from build123d import *

# Parameters (mm, degrees)
CHAMFER1_SIZE                                        = 2.5
CHAMFER2_SIZE                                        = 1.5
CSK_FOR_M10_COUNTERSUNK_FLAT_HEAD_SCREW1_D           = 11
CSK_FOR_M10_COUNTERSUNK_FLAT_HEAD_SCREW1_DEPTH       = 10.695266595
CSK_FOR_M10_COUNTERSUNK_FLAT_HEAD_SCREW1_CSINK_D     = 14
CSK_FOR_M10_COUNTERSUNK_FLAT_HEAD_SCREW1_CSINK_ANGLE = 90
CSK_FOR_M10_COUNTERSUNK_FLAT_HEAD_SCREW1_TIP         = 3.304733405
CSK_FOR_M10_COUNTERSUNK_FLAT_HEAD_SCREW2_D           = 11
CSK_FOR_M10_COUNTERSUNK_FLAT_HEAD_SCREW2_DEPTH       = 10.695266595
CSK_FOR_M10_COUNTERSUNK_FLAT_HEAD_SCREW2_CSINK_D     = 14
CSK_FOR_M10_COUNTERSUNK_FLAT_HEAD_SCREW2_CSINK_ANGLE = 90
CSK_FOR_M10_COUNTERSUNK_FLAT_HEAD_SCREW2_TIP         = 3.304733405


with BuildPart() as part:
    # Sketch1 → Revolve1 (revolve)
    with BuildSketch(Plane.XY):
        Polygon((0, 0), (0, 14.7), (17, 14.7), (17, 37.5), (109.5, 37.5), (109.5, 35), (128.5, 35), (141.5, 35), (141.5, 33), (257, 33), (257, 0), align=None)
    revolve(axis=Axis((0, 0, 0), (1, 0, 0)))

    # Chamfer1
    chamfer1_edges = [part.edges().sort_by_distance(p)[0] for p in [
        (17, -37.5, 0),
        (257, -33, 0),
    ]]
    chamfer(chamfer1_edges, length=CHAMFER1_SIZE)

    # Chamfer2
    chamfer2_edges = [part.edges().sort_by_distance(p)[0] for p in [
        (0, -14.7, 0),
    ]]
    chamfer(chamfer2_edges, length=CHAMFER2_SIZE)

    # CSK for M10 Countersunk Flat Head Screw1
    with Locations(Plane.ZY):
        with Locations((0, 0)):
            CounterSinkHole(CSK_FOR_M10_COUNTERSUNK_FLAT_HEAD_SCREW1_D / 2, CSK_FOR_M10_COUNTERSUNK_FLAT_HEAD_SCREW1_CSINK_D / 2, depth=CSK_FOR_M10_COUNTERSUNK_FLAT_HEAD_SCREW1_DEPTH, counter_sink_angle=CSK_FOR_M10_COUNTERSUNK_FLAT_HEAD_SCREW1_CSINK_ANGLE)
            with Locations((0, 0, -(CSK_FOR_M10_COUNTERSUNK_FLAT_HEAD_SCREW1_DEPTH + CSK_FOR_M10_COUNTERSUNK_FLAT_HEAD_SCREW1_TIP / 2))):  # 118° drill point
                Cone(0, CSK_FOR_M10_COUNTERSUNK_FLAT_HEAD_SCREW1_D / 2, CSK_FOR_M10_COUNTERSUNK_FLAT_HEAD_SCREW1_TIP, mode=Mode.SUBTRACT)

    # CSK for M10 Countersunk Flat Head Screw2
    with Locations(Plane(origin=(257, 0, 0), x_dir=(0, 0, -1), z_dir=(1, 0, 0))):
        with Locations((0, 0)):
            CounterSinkHole(CSK_FOR_M10_COUNTERSUNK_FLAT_HEAD_SCREW2_D / 2, CSK_FOR_M10_COUNTERSUNK_FLAT_HEAD_SCREW2_CSINK_D / 2, depth=CSK_FOR_M10_COUNTERSUNK_FLAT_HEAD_SCREW2_DEPTH, counter_sink_angle=CSK_FOR_M10_COUNTERSUNK_FLAT_HEAD_SCREW2_CSINK_ANGLE)
            with Locations((0, 0, -(CSK_FOR_M10_COUNTERSUNK_FLAT_HEAD_SCREW2_DEPTH + CSK_FOR_M10_COUNTERSUNK_FLAT_HEAD_SCREW2_TIP / 2))):  # 118° drill point
                Cone(0, CSK_FOR_M10_COUNTERSUNK_FLAT_HEAD_SCREW2_D / 2, CSK_FOR_M10_COUNTERSUNK_FLAT_HEAD_SCREW2_TIP, mode=Mode.SUBTRACT)


solid = part.part
Input: part model. Units: mm. Frame: model coordinates. A direction names the side the tool comes from. Give positions to 0.01 mm unless a question says otherwise; leave off trailing zeros. Write each loop counter-clockwise with the first axis right and the second up, starting at its lowest first coordinate (ties: lowest second). Pieces come first, ordered by that corner, then holes.
Q1. Material intervals for probe 1 along Z at (x, y) = (249, 0); probe 2 along Z at (x, y) = (7, 0); probe 3 along X at (y, z) = (26, -15), sorted ascending.
Q2. Section B-B, the plane x = 218. Output: boundary loops of the cut face in (y, z).
Q3. Set-up query: faces 4 (the face through (0, -6, -6)), 5 (the face through (9.36, -3.19, -14.35)), 6 (the face through (141.5, -23.5, 23.5)). Return all of +Z, -Z, +X, -X, +Y, -Y with unobstructed straight access to the full face (end or side cutting, diameter ignored); none if empty.
Q4. First-contact query: P1, Ø10, axis at y = 0, z = 0, coming from the -X side; P2, Ø3, axis at y = -16.5, z = 29.5, coming from the +X side; P3, Ø21, axis at y = 11.5, z = 15, coming from the -X side; P4, Ø8, axis at x = 128.5, z = -15.5, coming from the -Y side. Flat tips, straight axial feed; report the tip coordinate or a pass-through.
Q5. Pull-direction query (Y, two-part tool) for faces 1 (the face through (256.88, -6.64, -29.89)), 2 (the face through (257, -0.4, 7.2)), 3 (the face through (250.84, -5.37, -1.19)); classes: pulls with the +Y half, pulls with the -Y half, needs draft (parallel to the pull), parting line crosses it, or undercut.
Q6. Section A-A, the plane x = 27.5. Output: boundary loops of the cut face in (y, z).
Filled in:
1. probe 1: z = -33 to -5.5, 5.5 to 33
1. probe 2: z = -14.7 to -5.5, 5.5 to 14.7
1. probe 3: x = 17 to 257
2. outline: circle Ø66 at (0, 0)
3. face 4: +Z, -Z, -X, +Y, -Y
3. face 5: -X
3. face 6: +X
4. P1: stops at x = 11
4. P2: stops at x = 255.2
4. P3: stops at x = 0
4. P4: stops at y = -33.06
5. face 1: parting line crosses it
5. face 2: needs draft
5. face 3: undercut
6. outline: circle Ø75 at (0, 0)
